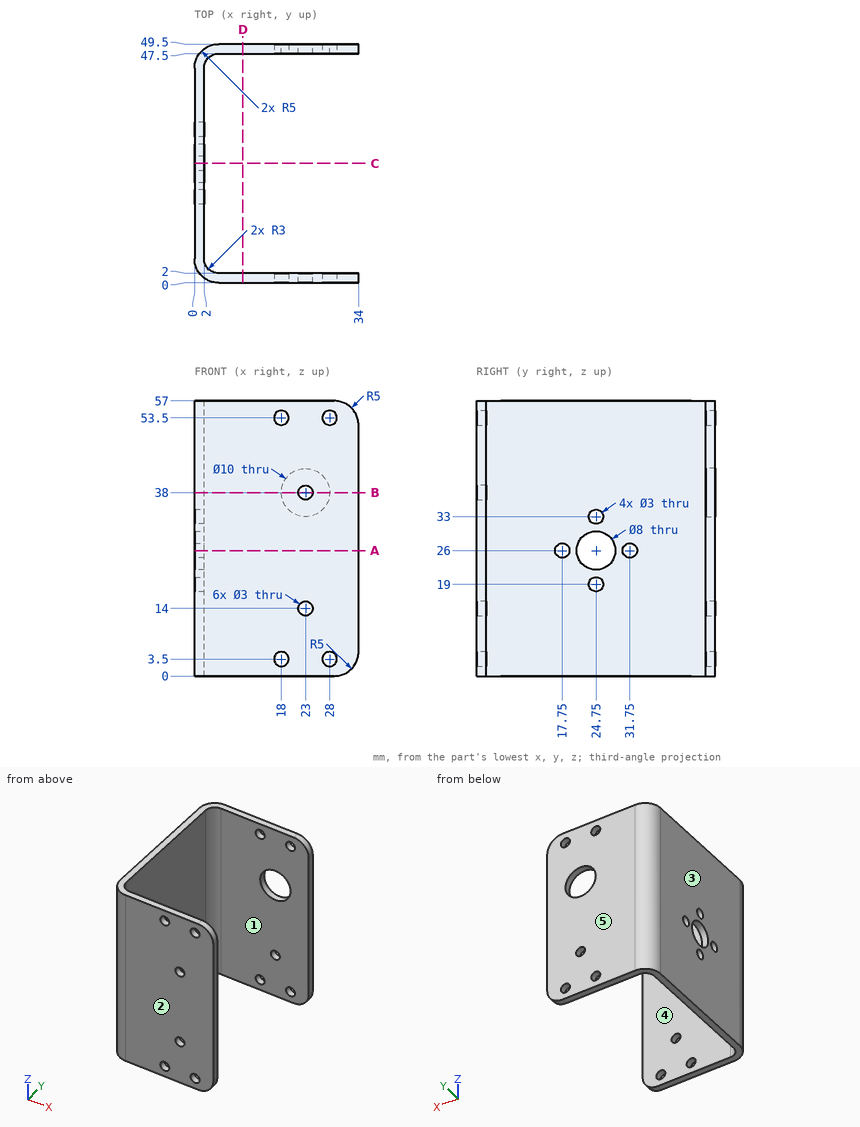
Could you check a few things on this drawing? It's one solid part, dimensions in mm from its lowest x, y, z. A direction names the side the tool comes from. Round coordinates to 2 decimals unless told otherwise and drop trailing zeros. Order: outer loops, then holes, each group sorted by start corner. A loop starts at its lowest first (then second) coordinate and runs counter-clockwise, first axis right, second up. Notation, with made-up numbers: M 77,50.25 L 107,50.25 A31 ccw 107,88.25 Z; hole C -33,1 d9. An arc over 180 degrees is marked long. Return JSON: item names as keys, results as strings. Group by question number.
1. I'm going to push a flat-ended pin straight in: pin 1 Ø3.5 at (y, z) = (17.75, 26) entering from +X. Where does the tip first touch, or does it pass through?
2. If we section it at D-D on x = 10: List the corners of the cut face in (y, z) for me.
3. On a 3-axis mill with a long thin cutter (end or side, diameter ignored), from which of +Z, -Z, +X, -X, +Y, -Y can I reach the whole of each face in a straight line? I mean the marked faces 4 and 5. Say none if no direction works.
4. If we section it at A-A on z = 26: List the corners of the cut face in (x, y) for me, then the cut area to 3 significant figures.
5. If we section it at B-B on z = 38: List the corners of the cut face in (x, y) for me.
6. If we mould it in two halves opening along Y, with no side actions, what happens to the marked faces 1, 2 and 3? For each: pulls with the +Y half, pulls with the -Y half, needs draft (parallel to the pull), parting line crosses it, or undercut.
7. Please list where these lines run through material, in increasing order: probe 1 along Y at (x, z) = (8, 7.5); probe 2 along X at (y, z) = (39.5, 29.5).
8. If we section it at C-C on y = 24.75: List the corners of the cut face in (x, z) for me.
Reply:
{
 "1": {"pin 1": "x = 2"},
 "2": {"outline": "M 0,0 L 2,0 L 2,57 L 0,57 Z; M 47.5,0 L 49.5,0 L 49.5,57 L 47.5,57 Z"},
 "3": {"face 4": "+Z, -Z, +X", "face 5": "+Z, -Z, +X, -X, +Y"},
 "4": {"outline": "M 0,5 A5 ccw 5,0 L 34,0 L 34,2 L 5,2 A3 cw 2,5 L 2,16.25 L 0,16.25 Z; M 0,19.25 L 2,19.25 L 2,20.75 L 0,20.75 Z; M 0,28.75 L 2,28.75 L 2,30.25 L 0,30.25 Z; M 0,33.25 L 2,33.25 L 2,44.5 A3 cw 5,47.5 L 34,47.5 L 34,49.5 L 5,49.5 A5 ccw 0,44.5 Z", "area": "192 mm^2"},
 "5": {"outline": "M 0,5 A5 ccw 5,0 L 21.5,0 L 21.5,2 L 5,2 A3 cw 2,5 L 2,44.5 A3 cw 5,47.5 L 18,47.5 L 18,49.5 L 5,49.5 A5 ccw 0,44.5 Z; M 24.5,0 L 34,0 L 34,2 L 24.5,2 Z; M 28,47.5 L 34,47.5 L 34,49.5 L 28,49.5 Z"},
 "6": {"face 1": "undercut", "face 2": "pulls with the -Y half", "face 3": "needs draft"},
 "7": {"probe 1": "0 to 2, 47.5 to 49.5", "probe 2": "0 to 2"},
 "8": {"outline": "M 0,0 L 2,0 L 2,17.5 L 0,17.5 Z; M 0,20.5 L 2,20.5 L 2,22 L 0,22 Z; M 0,30 L 2,30 L 2,31.5 L 0,31.5 Z; M 0,34.5 L 2,34.5 L 2,57 L 0,57 Z"}
}
